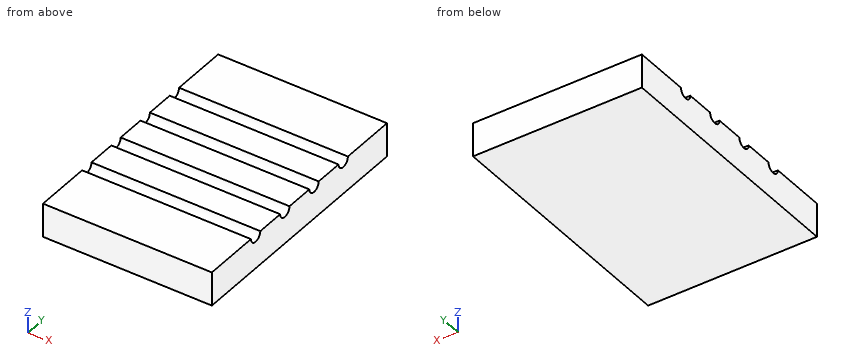
Autodesk Fusion 360 part; units mm, degrees
sketch "Sketch1" plane through (0, 0, 0) normal (0, 0, 1) x (1, 0, 0)
  line L0 (5, 7.5) -> (-5, 7.5)
  line L1 (-5, 7.5) -> (-5, -7.5)
  line L2 (-5, -7.5) -> (5, -7.5)
  line L3 (5, -7.5) -> (5, 7.5)
  line L4 (5, 7.5) -> (-5, -7.5) construction
  line L5 (-5, 7.5) -> (5, -7.5) construction
  dimension "d1" = 10
  dimension "d2" = 15
extrude "Extrude1" add sketch "Sketch1" along normal blind 3
sketch "Sketch2" plane through (5, 0, 0) normal (1, 0, 0) x (0, 1, 0)
  line L0 (-7.5, 0) -> (7.5, 0)
  line L1 (7.5, 0) -> (7.5, 3)
  line L2 (7.5, 3) -> (-7.5, 3)
  line L3 (-7.5, 3) -> (-7.5, 0)
  line L4 (0, 3) -> (5, 3) construction
  line L5 (5, 3) -> (3.75, 3) construction
  circle A0 centre (3.75, 3) radius 0.4
  line L6 (3.75, 3) -> (1.25, 3) construction
  circle A1 centre (1.25, 3) radius 0.4
  line L7 (0, 3) -> (0, 3.8715) construction
  circle A2 centre (-3.75, 3) radius 0.4
  circle A3 centre (-1.25, 3) radius 0.4
  dimension "d5" = 5
  dimension "d6" = 1.25
  dimension "d7" = 0.8
  dimension "d8" = 2.5
  dimension "d9" = 0.8
extrude "Extrude2" cut sketch "Sketch2" against normal blind 15 contours L2 A2 | L2 A0 | L2 A3 | L2 A1 picked at (-3.8463, 2.8894) picked at (3.8833, 2.7915) picked at (-1.1781, 2.8008) picked at (1.1833, 2.8845)
extrude "Extrude3" cut 1 faces at (-1.6667, 2.5, 0) along direction (0, 0, 1) blind 1
CAD build for the part. Positions are in the model's coordinates, mm. Coordinates: 2 decimals unless noted, no trailing zeros. Order: outer loops, then holes, each group sorted by start corner. A loop starts at its lowest first (then second) coordinate and runs counter-clockwise, first axis right, second up. Notation, with made-up numbers: (-32, 67.25) - (-14, 67.25) arc R25 cw to (-14, 89.25) - close; hole circle Ø8 at (49.5, 59). An arc over 180 degrees is marked (long way). Use a Markdown table: item, result. Add a question column.
(1) Saw through at B-B (x = 2.25). Give the cut face in (y, z).
(2) Saw through at C-C (y = 1.25). Give the cut face in (x, z), then the cut area to 3 significant figures.
(3) Drill centre lines: line 1 along Y through (x, z) = (-0.5, 2.7); line 2 along Y through (x, z) = (0.25, 2.85); line 3 along Z through (x, y) = (-2.5, -1.25). Where is each one in solid material? Low to high. Write a range as [from, to].
(4) Saw through at A-A (z = 2.75). Give the cut face in (x, y), then the cut area to 3 significant figures.
Solved:
| question | item | result |
|---|---|---|
| 1 | outline | (-7.5, 1) - (7.5, 1) - (7.5, 3) - (4.15, 3) arc R0.4 cw to (3.35, 3) - (1.65, 3) arc R0.4 cw to (0.85, 3) - (-0.85, 3) arc R0.4 cw to (-1.65, 3) - (-3.35, 3) arc R0.4 cw to (-4.15, 3) - (-7.5, 3) - close |
| 2 | outline | (-5, 1) - (5, 1) - (5, 2.6) - (-5, 2.6) - close |
| 2 | area | 16.0 mm² |
| 3 | line 1 | y = [-7.5, -4.01], [-3.49, -1.51], [-0.99, 0.99], [1.51, 3.49], [4.01, 7.5] |
| 3 | line 2 | y = [-7.5, -4.12], [-3.38, -1.62], [-0.88, 0.88], [1.62, 3.38], [4.12, 7.5] |
| 3 | line 3 | z = [1, 2.6] |
| 4 | outline | (-5, -7.5) - (5, -7.5) - (5, -4.06) - (-5, -4.06) - close; (-5, -3.44) - (5, -3.44) - (5, -1.56) - (-5, -1.56) - close; (-5, -0.94) - (5, -0.94) - (5, 0.94) - (-5, 0.94) - close; (-5, 1.56) - (5, 1.56) - (5, 3.44) - (-5, 3.44) - close; (-5, 4.06) - (5, 4.06) - (5, 7.5) - (-5, 7.5) - close |
| 4 | area | 125 mm² |
